The model under review builds one solid part; all positions refer to its coordinate system, in mm. Coordinates: 2 decimals unless noted, no trailing zeros. Write each loop counter-clockwise with the first axis right and the second up, starting at its lowest first coordinate (ties: lowest second). Pieces come first, ordered by that corner, then holes. Notation, with made-up numbers: (-27.75, 28.5) -> (7.25, 28.5) arc R14 cw to (7.25, 32.5) -> close; hole circle Ø7 at (-32, 3.25). An arc over 180 degrees is marked (long way). Write each question's results on one line, items separated by ' | '.
```python
from build123d import *

# Parameters (mm, degrees)
CHAMFER1_SIZE = 1
FILLET1_R     = 1


with BuildPart() as part:
    # Sketch1 → Revolve1 (revolve)
    with BuildSketch(Plane.XY, mode=Mode.PRIVATE) as revolve1_sk:
        Polygon((0, 8), (25, 8), (25, 10), (3, 10), (3, 13.5), (0, 13.5), align=None)
    revolve(revolve1_sk.sketch.rotate(Axis((0, 0, 0), (1, 0, 0)), 90), axis=Axis((0, 0, 0), (1, 0, 0)))

    # Chamfer1
    chamfer1_edges = [part.edges().sort_by_distance(p)[0] for p in [
        (0, 0, -13.5),
        (3, 0, -13.5),
        (25, 0, -10),
        (25, 0, -8),
        (0, 0, -8),
    ]]
    chamfer(chamfer1_edges, length=CHAMFER1_SIZE - 0.0001)  # a hair under: the kernel refuses the full size

    # Fillet1
    fillet1_edges = [part.edges().sort_by_distance(p)[0] for p in [
        (3, 0, -10),
    ]]
    fillet(fillet1_edges, radius=FILLET1_R)


solid = part.part
```
Q1. For line 1 (Y direction, x = 8, z = 0); line 2 (Z direction, x = 17, y = -7); line 3 (X direction, y = -5.25, z = 10.5), list the stretches that pass through material, from the lowest coordinate up. Write a range as from..to.
Solution:
line 1: -10..-8, 8..10 | line 2: -7.14..-3.87, 3.87..7.14 | line 3: 0..3
Q2. Draft analysis for pull direction Y (two halves, no side actions). For faces 1 (the flat face through (0, -9, -3)), 2 (the cylindrical face through (12.66, 7.81, -1.73)), 3 (the cylindrical face through (1.49, 13.18, -2.93)), state which applies: pulls with the +Y half, pulls with the -Y half, needs draft (parallel to the pull), parting line crosses it, or undercut.
Solution:
face 1: needs draft | face 2: undercut | face 3: parting line crosses it
Q3. Clearance check with flat-ended pins moving along their axes: P1, Ø5, axis at x = 8.5, z = 9.5, coming from the -Y side; P2, Ø8, axis at x = 5.5, y = -9.5, coming from the +Z side; P3, Ø3, axis at x = 10, z = 8.5, coming from the +Y side. State where each tip first meets the part, or that it passes through.
Solution:
P1: y = -7.14 | P2: z = 11.18 | P3: y = 7.14
Q4. Add section B-B (x = 22.5). Write out the cut boundary in (y, z), plus the area to 3 significant figures.
Solution:
outline: circle Ø20 at (0, 0); hole circle Ø16 at (0, 0) | area: 113 mm²
